Design review of the part built by this model. Coordinates are the model's own, in mm. Coordinates: 2 decimals unless noted, no trailing zeros. Loops run counter-clockwise (first coordinate to the right, second up) from the corner with the lowest first, then second, coordinate; pieces in that order, holes last. Notation, with made-up numbers: M 39.25,10.5 L 50.25,10.5 A11 ccw 50.25,19.5 Z; hole C 24.5,11.5 d5. An arc over 180 degrees is marked long. Answer as a JSON object with one key per item and string values. Group by question number.
1. Consider section B-B (x = -748). State the section outline as (y, z) points (3 decimals).
2. Consider section C-C (z = 346.5). State the section outline as (x, y) points (3 decimals).
3. To check wall thickness, follow probe 1 along X at (y, z) = (0.75, -139.7); probe 2 along Z at (x, y) = (-621, 2.9); probe 3 along X at (y, z) = (2.6, 371). State the ranges of each line that lie inside material, in increasing order.
4. Consider section A-A (y = 0.5). Count the separate pieces of the cut face and the enclosed holes in it, then the cut area to 3 significant figures.
from build123d import *

# Parameters (mm, degrees)
BOSS_EXTRUDE1_DEPTH = 3.175
SKETCH3_R           = 6.35
CUT_EXTRUDE1_DEPTH  = 4.175


with BuildPart() as part:
    # Sketch1 → Boss-Extrude1 (new body)
    with BuildSketch(Plane(origin=(0, 0, 0), x_dir=(1, 0, 0), z_dir=(0, 1, 0))):
        Polygon((0, 0), (0, 165.1), (-1073.15, 165.1), (-968.887028118, -490.232750074), align=None)
    extrude(amount=BOSS_EXTRUDE1_DEPTH)

    # Sketch3 → Cut-Extrude1 (cut, through all)
    with BuildSketch(Plane(origin=(0, 3.175, 0), x_dir=(1, 0, 0), z_dir=(0, 1, 0))):
        with Locations((-869.783056686, 139.7)):
            Circle(SKETCH3_R)
        with Locations((-666.583056686, 139.7)):
            Circle(SKETCH3_R)
        with Locations((-463.383056686, 139.7)):
            Circle(SKETCH3_R)
        with Locations((-260.183056686, 139.7)):
            Circle(SKETCH3_R)
        with Locations((-800.504721955, -376.569229128)):
            Circle(SKETCH3_R)
        with Locations((-619.192529558, -284.829767126)):
            Circle(SKETCH3_R)
        with Locations((-437.880337162, -193.090305124)):
            Circle(SKETCH3_R)
        with Locations((-256.568144766, -101.350843122)):
            Circle(SKETCH3_R)
    extrude(amount=-CUT_EXTRUDE1_DEPTH, mode=Mode.SUBTRACT)


solid = part.part
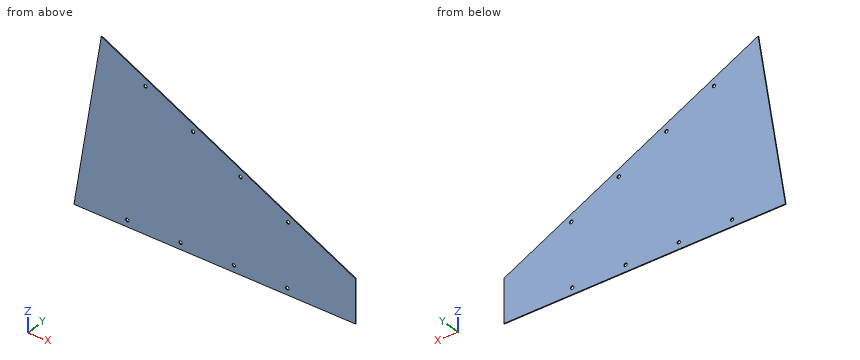
Findings below:
{
 "1": {"outline": "M 0,-165.1 L 3.175,-165.1 L 3.175,378.469 L 0,378.469 Z"},
 "2": {"outline": "M -991.755,0 L -684.816,0 L -684.816,3.175 L -991.755,3.175 Z"},
 "3": {"probe 1": "x = -1069.11 to -876.13, -863.43 to -672.93, -660.23 to -469.73, -457.03 to -266.53, -253.83 to 0", "probe 2": "z = -165.1 to 278.74, 290.92 to 314.21", "probe 3": "x = -987.86 to -803.56, -797.45 to -733.24"},
 "4": {"separate pieces": "1", "enclosed holes": "8", "area": "431,000 mm^2"}
}
